Can you work these out from the drawing? Everything is in mm from the part's minimum corner. A direction names the side the tool comes from. Round coordinates to 2 decimals unless told otherwise and drop trailing zeros. Write each loop counter-clockwise with the first axis right and the second up, starting at its lowest first coordinate (ties: lowest second). Pieces come first, ordered by that corner, then holes.
Q1. We'd pull the mould along X, two halves only. Please class the marked faces 3, 4 and 5: +X half, -X half, draft (parallel to the pull), parting line (faces both ways), or undercut.
Q2. If we section it at C-C (x = 54): Please give me the cut outline in (y, z) (1 decimal).
Q3. I'm going to push flat-ended pins straight in: pin 1 Ø4 at (x, y) = (59.5, 19.5) entering from -Z; pin 2 Ø1.7 at (x, y) = (75, 47.5) entering from +Z. Where does each tip first touch, or does it pass through?
Q4. If we section it at A-A (z = 3.75): Please give me the cut outline in (x, y) (1 decimal).
Q5. For the marked faces 1 and 2, which set-ups out of +Z, -Z, +X, -X, +Y, -Y let a thin tool reach every point of the face, with its end or its side?
Q6. Please list where these lines run through material, in increasing order: line 1 along X through (y, z) = (23.5, 11) (1 decimal); line 2 along Y through (x, z) = (21, 7.5) (1 decimal); line 3 along Z through (x, y) = (8, 40).
Q7. If we section it at B-B (y = 26.5): Please give me the cut outline in (x, z) (1 decimal).
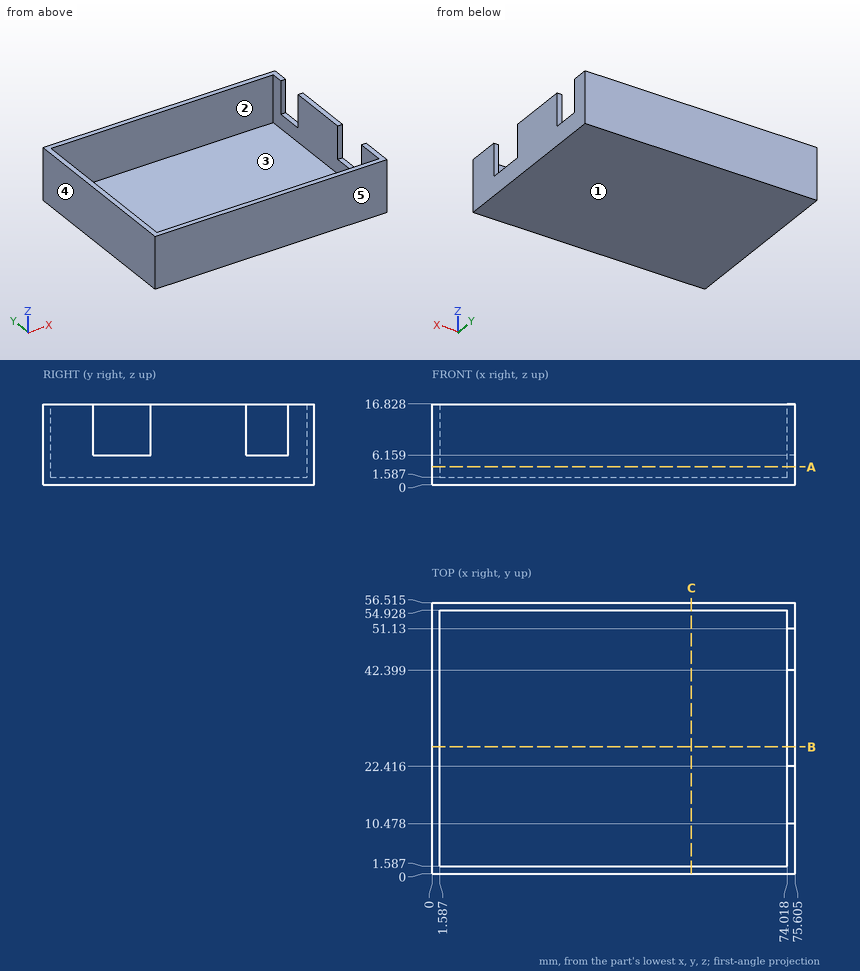
A:
1. face 3: undercut
1. face 4: -X half
1. face 5: draft
2. outline: (0, 0) - (56.5, 0) - (56.5, 16.8) - (54.9, 16.8) - (54.9, 1.6) - (1.6, 1.6) - (1.6, 16.8) - (0, 16.8) - close
3. pin 1: stops at z = 0
3. pin 2: stops at z = 6.16
4. outline: (0, 0) - (75.6, 0) - (75.6, 56.5) - (0, 56.5) - close; hole (1.6, 1.6) - (74, 1.6) - (74, 54.9) - (1.6, 54.9) - close
5. face 1: -Z, +X, -X, +Y, -Y
5. face 2: +Z
6. line 1: x = 0 to 1.6, 74 to 75.6
6. line 2: y = 0 to 1.6, 54.9 to 56.5
6. line 3: z = 0 to 1.59
7. outline: (0, 0) - (75.6, 0) - (75.6, 16.8) - (74, 16.8) - (74, 1.6) - (1.6, 1.6) - (1.6, 16.8) - (0, 16.8) - close
